For this review, use the dimensioned drawing (mm, ordinates from the lowest corner) and the shaded views. A direction names the side the tool comes from. Coordinates: 2 decimals unless noted, no trailing zeros. Order: outer loops, then holes, each group sorted by start corner. A loop starts at its lowest first (then second) coordinate and runs counter-clockwise, first axis right, second up. Notation, with made-up numbers: M 85,-18 L 107,-18 A30 cw 107,20 Z; hole C 80,7 d2. An arc over 180 degrees is marked long. Answer in a Markdown table with one row per item.
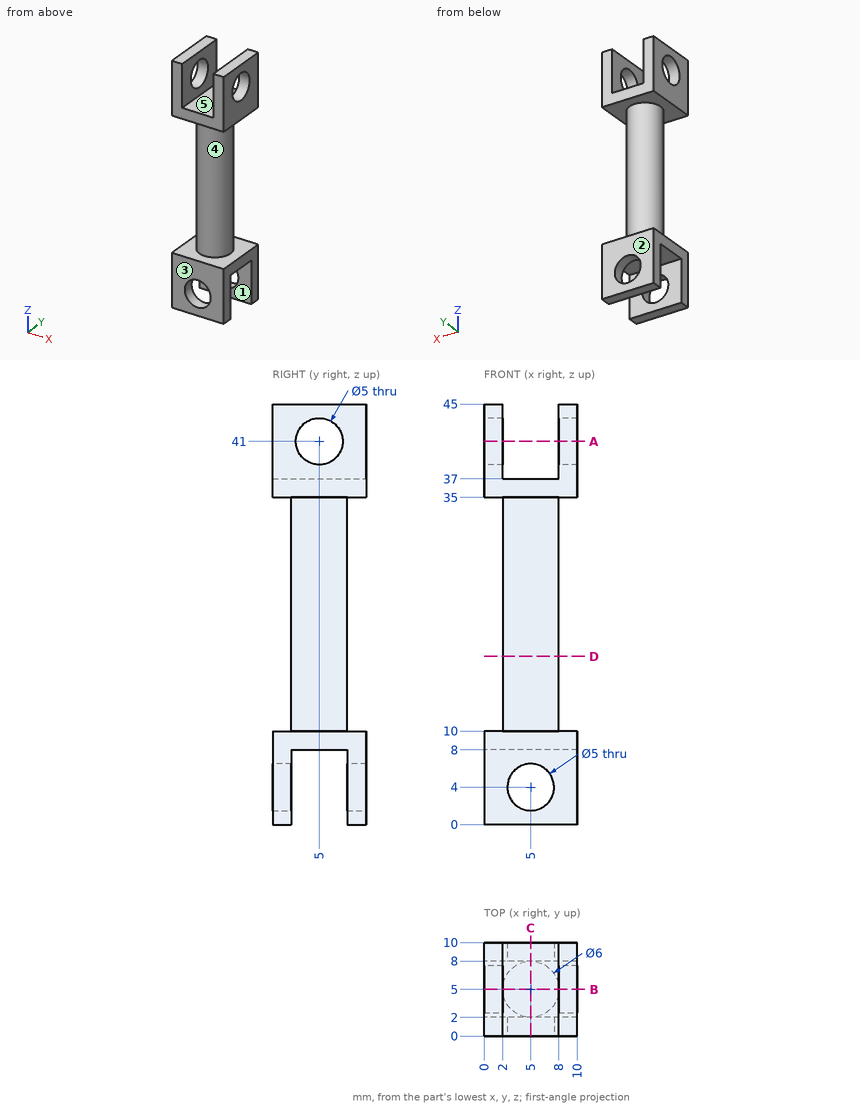
(1) Insertion check: pin 1 Ø1 at (x, y) = (2.5, 3) entering from -Z; pin 2 Ø1.5 at (x, z) = (8.5, 24.5) entering from +Y. Each pin has a flat end and moves straight along its axis. Give the tip position at first contact, or say it passes through.
Return value:
| item | result |
|---|---|
| pin 1 | stops at z = 8 |
| pin 2 | stops at y = 6.2 |
(2) Add section B-B, the plane y = 5. Give the boundary of the cut face in (x, z).
Return value:
| item | result |
|---|---|
| outline | M 0,8 L 10,8 L 10,10 L 8,10 L 8,35 L 10,35 L 10,38.5 L 8,38.5 L 8,37 L 2,37 L 2,38.5 L 0,38.5 L 0,35 L 2,35 L 2,10 L 0,10 Z; M 0,43.5 L 2,43.5 L 2,45 L 0,45 Z; M 8,43.5 L 10,43.5 L 10,45 L 8,45 Z |
(3) For line 1 along Z through (x, y) = (0.65, 5); line 2 along X through (y, z) = (1.5, 41), list the stretches that pass through material, from the lowest coordinate up. Write a range as from..to.
Return value:
| item | result |
|---|---|
| line 1 | z = 8..10, 35..38.5, 43.5..45 |
| line 2 | x = 0..2, 8..10 |
(4) Add section A-A, the plane z = 41. Give the boundary of the cut face in (x, y), and give its area (3 significant figures).
Return value:
| item | result |
|---|---|
| outline | M 0,0 L 2,0 L 2,2.5 L 0,2.5 Z; M 0,7.5 L 2,7.5 L 2,10 L 0,10 Z; M 8,0 L 10,0 L 10,2.5 L 8,2.5 Z; M 8,7.5 L 10,7.5 L 10,10 L 8,10 Z |
| area | 20.0 mm2 |
(5) Draft analysis for pull direction Z (two halves, no side actions). For the marked faces 3, 4 and 5, state which applies: pulls with the +Z half, pulls with the -Z half, needs draft (parallel to the pull), parting line crosses it, or undercut.
Return value:
| item | result |
|---|---|
| face 3 | needs draft |
| face 4 | undercut |
| face 5 | pulls with the +Z half |
(6) Add section D-D, the plane z = 18. Give the boundary of the cut face in (x, y), and give its area (3 significant figures).
Return value:
| item | result |
|---|---|
| outline | C 5,5 d6 |
| area | 28.3 mm2 |
(7) Add section C-C, the plane x = 5. Give the boundary of the cut face in (y, z).
Return value:
| item | result |
|---|---|
| outline | M 0,0 L 2,0 L 2,1.5 L 0,1.5 Z; M 0,6.5 L 2,6.5 L 2,8 L 8,8 L 8,6.5 L 10,6.5 L 10,10 L 8,10 L 8,35 L 10,35 L 10,37 L 0,37 L 0,35 L 2,35 L 2,10 L 0,10 Z; M 8,0 L 10,0 L 10,1.5 L 8,1.5 Z |
(8) For the marked faces 1 and 2, list the 3-axis set-ups (+Z, -Z, +X, -X, +Y, -Y) from which the entire face can be reached by the end or side of a thin tool; tool diameter is ignored.
Return value:
| item | result |
|---|---|
| face 1 | -Z, +X, -X |
| face 2 | +Z, -Z, +X, -X, +Y |
